Here's how the part is built. I have some questions about the finished solid (model axes, mm). A direction names the side the tool comes from. Round coordinates to 2 decimals unless told otherwise and drop trailing zeros. Write each loop counter-clockwise with the first axis right and the second up, starting at its lowest first coordinate (ties: lowest second). Pieces come first, ordered by that corner, then holes. Notation, with made-up numbers: (69.5, 60.25) -> (86.5, 60.25) arc R34 cw to (86.5, 92.25) -> close; hole circle Ø9 at (79, 89). An arc over 180 degrees is marked (long way). Answer in a Markdown table with one row per item. Add a question column.
from build123d import *

# Parameters (mm, degrees)
SKETCH1_W            = 42
SKETCH1_H            = 42
SKETCH1_R            = 11
BOSS_EXTRUDE1_DEPTH  = 1.5
M3_CLEARANCE_HOLE1_D = 3.2
SKETCH4_W            = 10
SKETCH4_H            = 28
BOSS_EXTRUDE2_DEPTH  = 3
SKETCH5_W            = 7
SKETCH5_H            = 0.7
BOSS_EXTRUDE3_DEPTH  = 3
FILLET1_R            = 1


with BuildPart() as part:
    # Sketch1 → Boss-Extrude1 (new, symmetric)
    with BuildSketch(Plane(origin=(0, 0, 0), x_dir=(1, 0, 0), z_dir=(0, 1, 0))):
        Rectangle(SKETCH1_W, SKETCH1_H)
        with Locations(Location((0, 0, 0), (0, 0, 270))):
            Circle(SKETCH1_R, mode=Mode.SUBTRACT)
    extrude(amount=BOSS_EXTRUDE1_DEPTH, both=True)

    # M3 Clearance Hole1 (through all)
    with Locations(Plane(origin=(0, 1.5, 0), x_dir=(1, 0, 0), z_dir=(0, 1, 0))):
        with Locations((-15.5, 15.5), (15.5, 15.5), (15.5, -15.5), (-15.5, -15.5)):
            Hole(M3_CLEARANCE_HOLE1_D / 2)

    # Sketch4 → Boss-Extrude2 (add)
    # profile 1 of 3: a face of its own
    with BuildSketch(Plane(origin=(0, 1.5, 0), x_dir=(1, 0, 0), z_dir=(0, 1, 0))):
        with BuildLine():
            Line((1.6, -24), (1.6, -28.7))
            Line((1.6, -28.7), (14, -28.7))
            Line((14, -28.7), (14, -21))
            Line((14, -21), (-14, -21))
            Line((-14, -21), (-14, -28.7))
            Line((-14, -28.7), (-1.6, -28.7))
            Line((-1.6, -28.7), (-1.6, -24))
            ThreePointArc((-1.6, -24), (0, -22.4), (1.6, -24))
        make_face()
    # profile 2 of 3: a face of its own
    with BuildSketch(Plane(origin=(0, 1.5, 0), x_dir=(1, 0, 0), z_dir=(0, 1, 0))):
        with BuildLine():
            Line((1.6, 28.7), (14, 28.7))
            Line((14, 28.7), (14, 21))
            Line((14, 21), (-14, 21))
            Line((-14, 21), (-14, 28.7))
            Line((-14, 28.7), (-1.6, 28.7))
            Line((-1.6, 28.7), (-1.6, 24))
            ThreePointArc((-1.6, 24), (0, 22.4), (1.6, 24))
            Line((1.6, 24), (1.6, 28.7))
        make_face()
    # profile 3 of 3: a face of its own
    with BuildSketch(Plane(origin=(0, 1.5, 0), x_dir=(1, 0, 0), z_dir=(0, 1, 0))):
        with Locations((26, 0)):
            Rectangle(SKETCH4_W, SKETCH4_H)
        with BuildLine():
            Line((27.6, 1.5), (27.6, -1.5))
            ThreePointArc((27.6, -1.5), (26, -3.1), (24.4, -1.5))
            Line((24.4, -1.5), (24.4, 1.5))
            ThreePointArc((24.4, 1.5), (26, 3.1), (27.6, 1.5))
        make_face(mode=Mode.SUBTRACT)
    extrude(amount=-BOSS_EXTRUDE2_DEPTH)

    # Sketch5 → Boss-Extrude3 (add)
    with BuildSketch(Plane(origin=(0, 1.5, 0), x_dir=(1, 0, 0), z_dir=(0, 1, 0))):
        Polygon((21, 14), (31, 14), (31, 21.7), (24, 21.7), (24, 28.7), (14, 28.7), (14, 21), (21, 21), align=None)
        Polygon((31, -14), (21, -14), (21, -21), (14, -21), (14, -28.7), (24, -28.7), (24, -21.7), (31, -21.7), align=None)
        with Locations((-17.5, -21.35)):
            Rectangle(SKETCH5_W, SKETCH5_H)
        with Locations((-17.5, 21.35)):
            Rectangle(SKETCH5_W, SKETCH5_H)
    extrude(amount=-BOSS_EXTRUDE3_DEPTH)

    # Fillet1
    fillet1_edges = [part.edges().sort_by_distance(p)[0] for p in [
        (-21, 0, 21.7),
        (31, 0, -21.7),
        (-21, 0, -21.7),
        (-14, 0, -21.7),
        (24, 0, -28.7),
        (24, 0, -21.7),
        (31, 0, 21.7),
        (24, 0, 21.7),
        (24, 0, 28.7),
        (-14, 0, 21.7),
        (-1.6, 0, 28.7),
        (-14, 0, 28.7),
        (1.6, 0, 28.7),
        (1.6, 0, -28.7),
        (-14, 0, -28.7),
        (-1.6, 0, -28.7),
    ]]
    fillet(fillet1_edges, radius=FILLET1_R)


solid = part.part
Item 1: For P1, Ø2.5, axis at x = 15.5, z = 15.5, coming from the +Y side; P2, Ø0.9, axis at y = -0.5, z = -25.5, coming from the -X side; P3, Ø1.5, axis at y = -0.5, z = -26, coming from the +X side, each with a flat end and sliding along its axis, tell me the tip position at first contact or that it passes through.
Item 2: If we section it at A-A on z = 0: Please give me the cut outline in (x, y).
Item 3: I need wall thicknesses on line 1 along Z through (x, y) = (-15.5, 0.5); line 2 along Z through (x, y) = (15.5, -0.15); line 3 along Z through (x, y) = (29, -0.9). Which ranges of each line are inside material? Lowest first, please. Write a range as from..to.
Item 4: If we mould it in two halves opening along Z, with no side actions, what happens to faces 5 (the flat face through (31, 0, 0)), 6 (the flat face through (28, 0, -21.7)), 7 (the flat face through (27, 0, 21.7)), 8 (the cylindrical face through (16.68, -0.02, -16.58))? For each: pulls with the +Z half, pulls with the -Z half, needs draft (parallel to the pull), parting line crosses it, or undercut.
Item 5: If we section it at C-C on z = 6.5: Please give me the cut outline in (x, y).
Item 6: On a 3-axis mill with a long thin cutter (end or side, diameter ignored), from which of +Z, -Z, +X, -X, +Y, -Y can I reach the whole of each face in a straight line? I mean faces 1 (the flat face through (-14, 0, 25)), 2 (the flat face through (24, 0, 25)), 3 (the flat face through (-18, 0, -21.7)), 4 (the cylindrical face through (26, 0, 3.1)). Say none if no direction works.
Item 7: If we section it at D-D on y = 0.6: Give the number of separate pieces and of enclosed holes in the cut face, then the cut area to 3 significant figures.
Item 8: If we section it at B-B on x = 0: Please give me the cut outline in (y, z), then the cut area to 3 significant figures.
Results list:
| question | item | result |
|---|---|---|
| 1 | P1 | through |
| 1 | P2 | x = -14 |
| 1 | P3 | x = 24 |
| 2 | outline | (-21, -1.5) -> (-11, -1.5) -> (-11, 1.5) -> (-21, 1.5) -> close; (11, -1.5) -> (24.4, -1.5) -> (24.4, 1.5) -> (11, 1.5) -> close; (27.6, -1.5) -> (31, -1.5) -> (31, 1.5) -> (27.6, 1.5) -> close |
| 3 | line 1 | -21.7..-17.1, -13.9..13.9, 17.1..21.7 |
| 3 | line 2 | -28.7..-17.1, -13.9..13.9, 17.1..28.7 |
| 3 | line 3 | -21.7..21.7 |
| 4 | face 5 | needs draft |
| 4 | face 6 | pulls with the -Z half |
| 4 | face 7 | pulls with the +Z half |
| 4 | face 8 | undercut |
| 5 | outline | (-21, -1.5) -> (-8.87, -1.5) -> (-8.87, 1.5) -> (-21, 1.5) -> close; (8.87, -1.5) -> (31, -1.5) -> (31, 1.5) -> (8.87, 1.5) -> close |
| 6 | face 1 | +Z, -X, +Y, -Y |
| 6 | face 2 | +Z, +X, +Y, -Y |
| 6 | face 3 | -Z, -X, +Y, -Y |
| 6 | face 4 | +Y, -Y |
| 7 | separate pieces | 1 |
| 7 | enclosed holes | 6 |
| 7 | area | 2,320 mm² |
| 8 | outline | (-1.5, -22.4) -> (1.5, -22.4) -> (1.5, -11) -> (-1.5, -11) -> close; (-1.5, 11) -> (1.5, 11) -> (1.5, 22.4) -> (-1.5, 22.4) -> close |
| 8 | area | 68.4 mm² |
